Input: part model. Units: mm. Frame: model coordinates. A direction names the side the tool comes from. Give positions to 0.01 mm unless a question says otherwise; leave off trailing zeros. Write each loop counter-clockwise with the first axis right and the second up, starting at its lowest first coordinate (ties: lowest second). Pieces come first, ordered by that corner, then holes. Notation, with made-up numbers: (67.25, 41) -> (77.25, 41) arc R23 ccw to (77.25, 62) -> close; hole circle Ø6 at (69, 13). An arc over 180 degrees is marked (long way). Return JSON: item names as keys, results as strings. Group by question number.
Item 1: Section A-A, the plane x = 53. Return loops of the section in (y, z), then the cut area to 3 significant figures.
Item 2: Section C-C, the plane y = 6. Return loops of the section in (x, z), then the cut area to 3 significant figures.
Item 3: Section B-B, the plane y = 13. Return loops of the section in (x, z).
Item 4: Line query: line 1 (X direction, y = 7.5, z = 2.2); line 2 (Y direction, x = 6.5, z = 1.3); line 3 (X direction, y = 6, z = 5.75). Output: solid intervals per line, ascending. Write a range as [from, to].
Item 5: Pin query (flat end, axial travel): P1, Ø3, axis at x = 53, y = 12, coming from the +Z side; P2, Ø0.8, axis at y = 3.5, z = 2.5, coming from the -X side; P3, Ø0.5, axis at y = 7, z = 4.5, coming from the -X side; P4, Ø1.8, axis at x = 16.5, z = 4.5, coming from the +Y side. Return the tip coordinate at first contact, or that it passes through.
Item 6: Set-up query: faces 1 (the face through (45, 5, 6)), 2 (the face through (35, 5, 5)). Return all of +Z, -Z, +X, -X, +Y, -Y with unobstructed straight access to the full face (end or side cutting, diameter ignored); none if empty.
Item 7: Section D-D, the plane z = 1.3. Return loops of the section in (x, y), then the cut area to 3 significant figures.
from build123d import *

# Parameters (mm, degrees)
SKETCH1_W        = 50
SKETCH1_H        = 10
F_2MM_DEPTH      = 2
SKETCH2_W        = 40
SKETCH2_H        = 10
F_3MM_DEPTH      = 1
SKETCH3_W        = 30
SKETCH3_H        = 10
F_4MM_DEPTH      = 1
SKETCH4_W        = 20
SKETCH4_H        = 10
F_5MM_DEPTH      = 1
SKETCH5_W        = 10
SKETCH5_H        = 10
F_6MM_DEPTH      = 1
SKETCH6_R        = 5
PRINT_EARS_DEPTH = 0.3


with BuildPart() as part:
    # Sketch1 → 2mm (new body)
    with BuildSketch(Plane.XY):
        with Locations((25, 5)):
            Rectangle(SKETCH1_W, SKETCH1_H)
    extrude(amount=F_2MM_DEPTH)

    # Sketch2 → 3mm (add)
    with BuildSketch(Plane.XY.offset(2)):
        with Locations((30, 5)):
            Rectangle(SKETCH2_W, SKETCH2_H)
    extrude(amount=F_3MM_DEPTH)

    # Sketch3 → 4mm (add)
    with BuildSketch(Plane.XY.offset(3)):
        with Locations((35, 5)):
            Rectangle(SKETCH3_W, SKETCH3_H)
    extrude(amount=F_4MM_DEPTH)

    # Sketch4 → 5mm (add)
    with BuildSketch(Plane.XY.offset(4)):
        with Locations((40, 5)):
            Rectangle(SKETCH4_W, SKETCH4_H)
    extrude(amount=F_5MM_DEPTH)

    # Sketch5 → 6mm (add)
    with BuildSketch(Plane.XY.offset(5)):
        with Locations((45, 5)):
            Rectangle(SKETCH5_W, SKETCH5_H)
    extrude(amount=F_6MM_DEPTH)

    # Sketch6 → Print ears (add)
    with BuildSketch(Plane(origin=(0, 0, 0), x_dir=(-1, 0, 0), z_dir=(0, 0, -1))):
        with Locations((3, -3)):
            Circle(SKETCH6_R)
        with Locations((3, 13)):
            Circle(SKETCH6_R)
        with Locations((-53, 13)):
            Circle(SKETCH6_R)
        with Locations((-53, -3)):
            Circle(SKETCH6_R)
    extrude(amount=-PRINT_EARS_DEPTH)


solid = part.part
Answer below:
{
 "1": {"outline": "(-8, 0) -> (2, 0) -> (2, 0.3) -> (-8, 0.3) -> close; (8, 0) -> (18, 0) -> (18, 0.3) -> (8, 0.3) -> close", "area": "6.00 mm2"},
 "2": {"outline": "(0, 0) -> (50, 0) -> (50, 6) -> (40, 6) -> (40, 5) -> (30, 5) -> (30, 4) -> (20, 4) -> (20, 3) -> (10, 3) -> (10, 2) -> (0, 2) -> close", "area": "200 mm2"},
 "3": {"outline": "(-8, 0) -> (2, 0) -> (2, 0.3) -> (-8, 0.3) -> close; (48, 0) -> (58, 0) -> (58, 0.3) -> (48, 0.3) -> close"},
 "4": {"line 1": "x = [10, 50]", "line 2": "y = [0, 10]", "line 3": "x = [40, 50]"},
 "5": {"P1": "stops at z = 0.3", "P2": "stops at x = 10", "P3": "stops at x = 30", "P4": "passes through"},
 "6": {"face 1": "+Z, +X, -X, +Y, -Y", "face 2": "+Z, -X, +Y, -Y"},
 "7": {"outline": "(0, 0) -> (50, 0) -> (50, 10) -> (0, 10) -> close", "area": "500 mm2"}
}
